Autodesk Inventor part; units mm, degrees
ref_plane "YZ Plane" through (0, 0, 0) normal (1, 0, 0) x (0, 1, 0)
ref_plane "XZ Plane" through (0, 0, 0) normal (0, 1, 0) x (-1, 0, 0)
ref_plane "XY Plane" through (0, 0, 0) normal (0, 0, 1) x (1, 0, 0)
sketch "Sketch1" plane through (0, 0, 0) normal (0, 1, 0) x (-1, 0, 0)
  line L0 (-225, 302.5) -> (225, 302.5)
  line L1 (225, 302.5) -> (225, -302.5)
  line L2 (225, -302.5) -> (-225, -302.5)
  line L3 (-225, -302.5) -> (-225, 302.5)
  line L4 (-225, 302.5) -> (225, -302.5) construction
  line L5 (225, 302.5) -> (-225, -302.5) construction
  line L6 (-219, 296.5) -> (219, 296.5)
  line L7 (219, 296.5) -> (219, -296.5)
  line L8 (219, -296.5) -> (-219, -296.5)
  line L9 (-219, -296.5) -> (-219, 296.5)
  line L10 (-219, 296.5) -> (219, -296.5) construction
  line L11 (219, 296.5) -> (-219, -296.5) construction
  line L12 (-219, 296.5) -> (-225, 296.5)
  line L13 (-219, 296.5) -> (-213, 296.5) construction
  line L14 (-219, -296.5) -> (-225, -296.5)
  line L15 (-219, -296.5) -> (-213, -296.5) construction
  point P0 (0, 0)
  dimension "d0" = 450
  dimension "d1" = 605
  dimension "d2" = 438
  dimension "d3" = 593
  dimension "d4" = 6
  dimension "d5" = 180
  dimension "d6" = 6
  dimension "d7" = 180
extrude "Extrusion1" add sketch "Sketch1" along normal blind 635 contours L0 L1 L2 L3 L14 L8 L7 L6 L12
sketch "Sketch2" plane through (-219, 0, -296.5) normal (0, 0, 1) x (1, 0, 0)
  line L0 (0, 635) -> (444, 635)
  line L1 (444, 0) -> (444, 635)
  line L2 (0, 635) -> (444, 635)
  line L3 (444, 635) -> (444, 623)
  line L4 (444, 623) -> (0, 623)
  line L5 (0, 623) -> (0, 635)
  line L6 (0, 0) -> (444, 0)
  line L7 (444, 0) -> (444, 12)
  line L8 (444, 12) -> (0, 12)
  line L9 (0, 12) -> (0, 0)
  point P0 (219, 0)
  dimension "d10" = 12
  dimension "d13" = 12
extrude "Extrusion2" add sketch "Sketch2" along normal up to surface (593 mm away)
sketch "Sketch3" plane through (0, 635, 0) normal (0, 1, 0) x (1, 0, 0)
  circle A0 centre (-73, -177.5) radius 80
  line L0 (-225, 302.5) -> (-225, -302.5)
  line L1 (-225, -302.5) -> (225, -302.5)
  circle A1 centre (-125, 202.5) radius 37.5
  line L2 (225, 302.5) -> (-225, 302.5)
  line L3 (-213, -57.5) -> (-143, -57.5)
  line L4 (-143, -57.5) -> (-143, 12.5)
  line L5 (-143, 12.5) -> (-213, 12.5)
  line L6 (-213, 12.5) -> (-213, -57.5)
  line L7 (-213, -57.5) -> (-143, 12.5) construction
  line L8 (-143, -57.5) -> (-213, 12.5) construction
  circle A2 centre (15, -52.5) radius 55
  line L9 (225, -302.5) -> (225, 302.5)
  line L10 (-53, 85.5) -> (-213, 85.5)
  line L11 (-213, 85.5) -> (-213, 290.5)
  line L12 (-213, 290.5) -> (-53, 290.5)
  line L13 (-53, 290.5) -> (-53, 85.5)
  line L14 (-53, 85.5) -> (-213, 290.5) construction
  line L15 (-213, 85.5) -> (-53, 290.5) construction
  point P0 (0, 0)
  point P1 (-178, -22.5)
  point P2 (-133, 188)
  dimension "d14" = 160
  dimension "d15" = 152
  dimension "d16" = 125
  dimension "d17" = 75
  dimension "d18" = 100
  dimension "d19" = 100
  dimension "d20" = 325
  dimension "d21" = 47
  dimension "d22" = 70
  dimension "d23" = 70
  dimension "d24" = 110
  dimension "d25" = 210
  dimension "d26" = 250
  dimension "d37" = 205
  dimension "d38" = 160
  dimension "d39" = 12
  dimension "d40" = 12
extrude "Extrusion3" cut sketch "Sketch3" against normal blind 100 contours A0 | A1 | L6 L5 L4 L3 | A2 | L10 L11 L12 L13
sketch "Sketch4" plane through (225, 0, -302.5) normal (0, 0, -1) x (-1, 0, 0)
  line L0 (255, 587.5) -> (410, 587.5)
  line L1 (410, 587.5) -> (410, 502.5)
  line L2 (410, 502.5) -> (255, 502.5)
  line L3 (255, 502.5) -> (255, 587.5)
  line L4 (255, 587.5) -> (410, 502.5) construction
  line L5 (410, 587.5) -> (255, 502.5) construction
  line L6 (450, 0) -> (450, 635)
  line L7 (0, 635) -> (450, 635)
  point P0 (225, 0)
  point P1 (332.5, 545)
  dimension "d31" = 155
  dimension "d32" = 85
  dimension "d33" = 40
  dimension "d34" = 90
extrude "Extrusion4" cut sketch "Sketch4" against normal blind 100
sketch "Sketch5" plane through (-219, 12, 296.5) normal (1, 0, 0) x (0, 0, -1)
  line L0 (22.5, 561) -> (332.5, 561)
  line L1 (332.5, 561) -> (332.5, 529)
  line L2 (332.5, 529) -> (22.5, 529)
  line L3 (22.5, 529) -> (22.5, 561)
  line L4 (22.5, 561) -> (332.5, 529) construction
  line L5 (332.5, 561) -> (22.5, 529) construction
  line L6 (0, 0) -> (0, 611)
  line L7 (593, 611) -> (0, 611)
  point P0 (296.5, -12)
  point P1 (177.5, 545)
  dimension "d41" = 22.5
  dimension "d42" = 310
  dimension "d43" = 32
  dimension "d44" = 82
extrude "Extrusion5" add sketch "Sketch5" along normal blind 260
sketch "Sketch6" plane through (-219, 12, 296.5) normal (1, 0, 0) x (0, 0, -1)
  line L0 (423, 458) -> (593, 458)
  line L1 (593, 458) -> (593, 446)
  line L2 (593, 446) -> (423, 446)
  line L3 (423, 446) -> (423, 458)
  line L4 (423, 458) -> (593, 446) construction
  line L5 (593, 458) -> (423, 446) construction
  line L6 (593, 611) -> (0, 611)
  line L7 (593, 0) -> (593, 611)
  point P0 (296.5, -12)
  point P1 (508, 452)
  dimension "d47" = 170
  dimension "d48" = 12
  dimension "d49" = 165
  dimension "d50" = 0
extrude "Extrusion6" add sketch "Sketch6" along normal blind 220
sketch "Sketch7" plane through (-219, 12, -296.5) normal (0, 1, 0) x (1, 0, 0)
  circle A0 centre (119, -353) radius 50
  line L0 (444, 0) -> (444, -593)
  line L1 (444, -593) -> (0, -593)
  point P0 (219, -296.5)
  dimension "d53" = 100
  dimension "d54" = 325
  dimension "d55" = 240
extrude "Extrusion7" add sketch "Sketch7" along normal blind 10
sketch "Sketch8" plane through (-100, 22, 56.5) normal (0, 1, 0) x (1, 0, 0)
  circle A0 centre (0, 0) radius 15
  point P0 (100, 56.5)
  dimension "d58" = 30
extrude "Extrusion8" add sketch "Sketch8" along normal blind 327
sketch "Sketch9" plane through (-100, 349, 56.5) normal (0, 1, 0) x (1, 0, 0)
  line L0 (97.5, -90) -> (-92.5, -90)
  line L1 (-92.5, -90) -> (-92.5, 95)
  line L2 (-92.5, 95) -> (97.5, 95)
  line L3 (97.5, 95) -> (97.5, -90)
  line L4 (97.5, -90) -> (-92.5, 95) construction
  line L5 (-92.5, -90) -> (97.5, 95) construction
  point P0 (100, 56.5)
  point P1 (2.5, 2.5)
  dimension "d61" = 190
  dimension "d62" = 185
extrude "Extrusion9" add sketch "Sketch9" along normal blind 3
properties part number "Outer Casing"
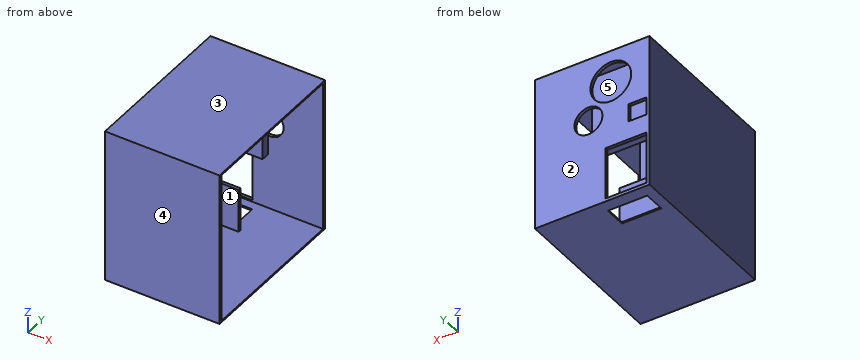
Input: part model. Units: mm. Frame: model coordinates. Face numbers are marked on the shaded views. A direction names the side the tool comes from. Round coordinates to 2 decimals unless told otherwise and drop trailing zeros. Loops run counter-clockwise (first coordinate to the right, second up) from the corner with the lowest first, then second, coordinate; pieces in that order, holes last. Notation, with made-up numbers: (46, 29) -> (79, 29) arc R22 cw to (79, 46) -> close; hole circle Ø11 at (70.25, -25.5). An arc over 180 degrees is marked (long way). Write each question's results on one line, items separated by ' | '.
1. Section C-C (z = 265.5). Return loops of the section in (x, y), and give its area (3 significant figures).
Geometry results:
outline: (-225, 0) -> (225, 0) -> (225, 12) -> (-219, 12) -> (-219, 541) -> (41, 541) -> (41, 573) -> (-219, 573) -> (-219, 623) -> (225, 623) -> (225, 635) -> (-225, 635) -> close | area: 22,800 mm2
2. Section B-B (x = 15). Return loops of the section in (y, z), and give its area (3 significant figures).
Geometry results:
outline: (0, -302.5) -> (635, -302.5) -> (635, -2.5) -> (623, -2.5) -> (623, -296.5) -> (12, -296.5) -> (12, 296.5) -> (623, 296.5) -> (623, 107.5) -> (635, 107.5) -> (635, 302.5) -> (0, 302.5) -> close; (541, -36) -> (573, -36) -> (573, 274) -> (541, 274) -> close | area: 30,500 mm2
3. First-contact query: P1, Ø3.5, axis at y = 351, z = 84, coming from the +X side. Flat tip, straight axial feed; report the tip coordinate or a pass-through.
Geometry results:
P1: x = -2.5
4. Section D-D (x = 139). Return loops of the section in (y, z), and give its area (3 significant figures).
Geometry results:
outline: (0, -302.5) -> (635, -302.5) -> (635, 302.5) -> (0, 302.5) -> close; hole (12, -296.5) -> (623, -296.5) -> (623, 296.5) -> (12, 296.5) -> close | area: 21,900 mm2
5. Mould query, pull axis Z, two halves, no side actions, for the marked faces 1, 2 and 3. Classes: +Z half, -Z half, draft (parallel to the pull), parting line (faces both ways), or undercut.
Geometry results:
face 1: undercut | face 2: draft | face 3: +Z half
6. Set-up query: the marked faces 4 and 5. Return all of +Z, -Z, +X, -X, +Y, -Y with unobstructed straight access to the full face (end or side cutting, diameter ignored); none if empty.
Geometry results:
face 4: +Z, -Z, +X, -X, -Y | face 5: +X
7. Ray query, line 1 (Y direction, x = -138.5, z = 43.5); line 2 (X direction, y = 628.5, z = 52.5); line 3 (Z direction, x = -73, y = 632.25). Return the intervals inside material, ascending. Write a range as from..to.
Geometry results:
line 1: 0..22, 349..352, 541..573, 623..635 | line 2: -225..-213, -143..-40, 70..225 | line 3: -302.5..-290.5, -85.5..97.5, 257.5..302.5
8. Section A-A (y = 557). Return loops of the section in (x, z), and give its area (3 significant figures).
Geometry results:
outline: (-225, -302.5) -> (-185, -302.5) -> (-185, -296.5) -> (-219, -296.5) -> (-219, -36) -> (41, -36) -> (41, 274) -> (-219, 274) -> (-219, 296.5) -> (225, 296.5) -> (225, 302.5) -> (-225, 302.5) -> close; (-30, -302.5) -> (225, -302.5) -> (225, -296.5) -> (-30, -296.5) -> close | area: 88,600 mm2
